Design review of the part shown in the three views and the two pictorial views. Dimensions are in mm from the part's minimum x, y and z. Coordinates: 2 decimals unless noted, no trailing zeros. Loops run counter-clockwise (first coordinate to the right, second up) from the corner with the lowest first, then second, coordinate; pieces in that order, holes last. Notation, with made-up numbers: (5.25, -18) -> (25.25, -18) arc R18 cw to (25.25, 2) -> close; hole circle Ø9 at (-16, 7.25). An arc over 180 degrees is marked (long way). Use a Markdown table: item, result. Add a question column.
Q1. Draft analysis for pull direction X (two halves, no side actions). For the marked faces 1, 2 and 3, state which applies: pulls with the +X half, pulls with the -X half, needs draft (parallel to the pull), parting line crosses it, or undercut.
Q2. Clearance check with flat-ended pins moving along their axes: pin 1 Ø0.7 at (y, z) = (1.5, 2) entering from +X; pin 2 Ø1.5 at (x, y) = (2, 1.5) entering from -Z; pin 3 Ø0.7 at (x, z) = (3.5, 2) entering from -Y; pin 4 Ø0.5 at (x, z) = (4, 8) entering from +Y. State where each tip first meets the part, or that it passes through.
Q3. Take a section at B-B on y = 0.2. Write out the cut boundary in (x, z).
Q4. Take a section at A-A on z = 9.5. Write out the cut boundary in (x, y).
Q5. Take a section at C-C on x = 3.75. Write out the cut boundary in (y, z).
Q6. Take a section at D-D on z = 5. Write out the cut boundary in (x, y), plus the area to 3 significant figures.
Q7. For probe 1 along X at (y, z) = (1.2, 8.25); probe 2 along Z at (x, y) = (2.2, 1.6); probe 3 along X at (y, z) = (2.2, 4.25) (1 decimal), list the stretches that pass through material, from the lowest coordinate up.
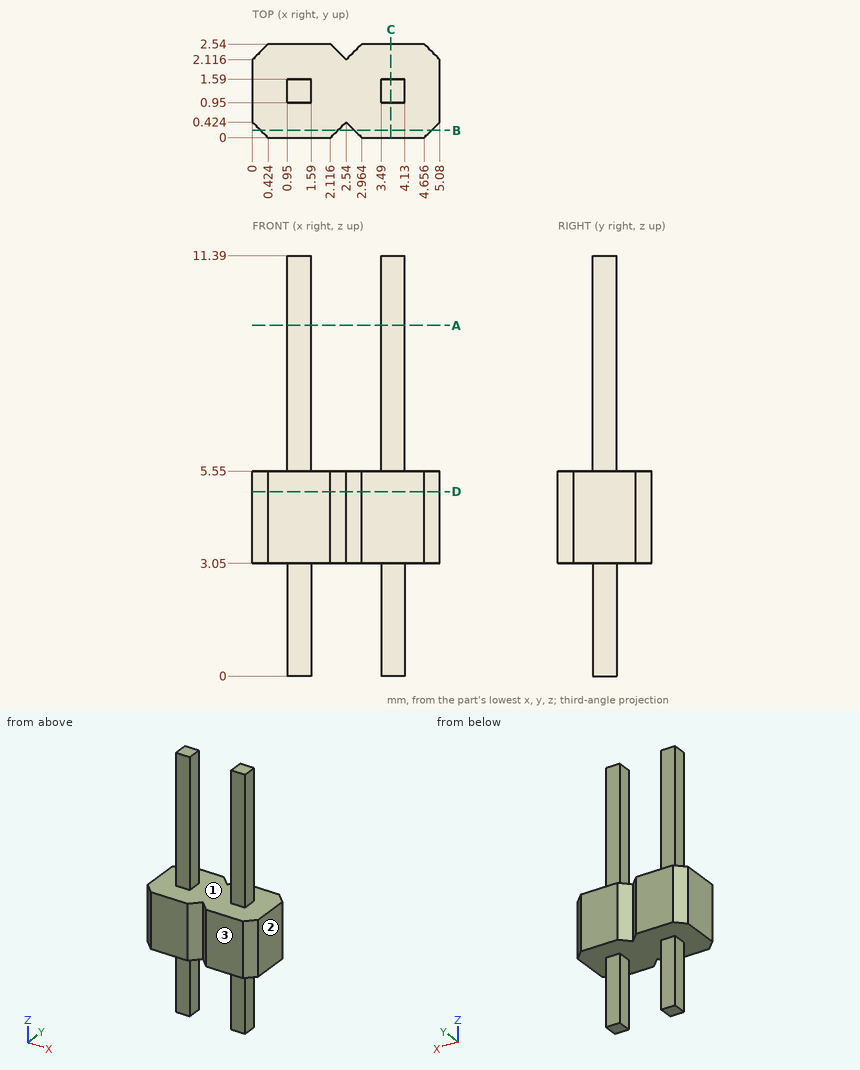
Answer list:
| question | item | result |
|---|---|---|
| 1 | face 1 | undercut |
| 1 | face 2 | pulls with the +X half |
| 1 | face 3 | needs draft |
| 2 | pin 1 | x = 4.13 |
| 2 | pin 2 | z = 0 |
| 2 | pin 3 | y = 0.95 |
| 2 | pin 4 | y = 1.59 |
| 3 | outline | (0.22, 3.05) -> (2.32, 3.05) -> (2.32, 5.55) -> (0.22, 5.55) -> close; (2.76, 3.05) -> (4.86, 3.05) -> (4.86, 5.55) -> (2.76, 5.55) -> close |
| 4 | outline | (0.95, 0.95) -> (1.59, 0.95) -> (1.59, 1.59) -> (0.95, 1.59) -> close; (3.49, 0.95) -> (4.13, 0.95) -> (4.13, 1.59) -> (3.49, 1.59) -> close |
| 5 | outline | (0, 3.05) -> (0.95, 3.05) -> (0.95, 0) -> (1.59, 0) -> (1.59, 3.05) -> (2.54, 3.05) -> (2.54, 5.55) -> (1.59, 5.55) -> (1.59, 11.39) -> (0.95, 11.39) -> (0.95, 5.55) -> (0, 5.55) -> close |
| 6 | outline | (0, 0.42) -> (0.42, 0) -> (2.12, 0) -> (2.54, 0.42) -> (2.96, 0) -> (4.66, 0) -> (5.08, 0.42) -> (5.08, 2.12) -> (4.66, 2.54) -> (2.96, 2.54) -> (2.54, 2.12) -> (2.12, 2.54) -> (0.42, 2.54) -> (0, 2.12) -> close |
| 6 | area | 12.2 mm² |
| 7 | probe 1 | 0.95 to 1.59, 3.49 to 4.13 |
| 7 | probe 2 | 3.05 to 5.55 |
| 7 | probe 3 | 0.1 to 2.5, 2.6 to 5 |
